For this review, take the finished solid that the model builds, in its own axes (mm). Round coordinates to 2 decimals unless told otherwise and drop trailing zeros. Order: outer loops, then holes, each group sorted by start corner. A loop starts at its lowest first (then second) coordinate and runs counter-clockwise, first axis right, second up. Notation, with made-up numbers: (38.5, 35) -> (68.5, 35) arc R17 cw to (68.5, 66) -> close; hole circle Ø8 at (-8.75, 74). An arc over 180 degrees is marked (long way). Answer in a Markdown table with one row per item.
```python
from build123d import *

# Parameters (mm, degrees)
SKETCH1_R           = 2.25
BOSS_EXTRUDE1_DEPTH = 5


with BuildPart() as part:
    # Sketch1 → Boss-Extrude1 (new body)
    with BuildSketch(Plane.XZ.offset(63)):
        with BuildLine():
            Line((8.181928414, -16.605718064), (17.802171103, -33.691169181))
            ThreePointArc((17.802171103, -33.691169181), (18.572370652, -35.426303597), (19.000782012, -37.275725803))
            ThreePointArc((19.000782012, -37.275725803), (24.55776359, -40.047666423), (25.069213931, -33.85879596))
            ThreePointArc((25.069213931, -33.85879596), (23.710027, -32.533462163), (22.625796475, -30.975148024))
            Line((22.625796475, -30.975148024), (13.005553786, -13.889696907))
            ThreePointArc((13.005553786, -13.889696907), (12.235354237, -12.15456249), (11.806942877, -10.305140285))
            ThreePointArc((11.806942877, -10.305140285), (6.249961299, -7.533199664), (5.738510958, -13.722070128))
            ThreePointArc((5.738510958, -13.722070128), (7.097697889, -15.047403925), (8.181928414, -16.605718064))
        make_face()
        with Locations((22.71787829, -36.780049236)):
            Circle(SKETCH1_R, mode=Mode.SUBTRACT)
        with Locations((8.089846599, -10.800816852)):
            Circle(SKETCH1_R, mode=Mode.SUBTRACT)
    extrude(amount=-BOSS_EXTRUDE1_DEPTH)


solid = part.part
```
Q1. The part is to be moulded in two halves that separate along X. For faces 1 (the face through (17.88, -60.54, -22.55)), 2 (the face through (7.08, -60.535, -15.027)), 3 (the face through (20.932, -60.535, -38.149)), say which applies: +X half, -X half, draft (parallel to the pull), parting line (faces both ways), or undercut.
Answer key:
| item | result |
|---|---|
| face 1 | +X half |
| face 2 | -X half |
| face 3 | undercut |
Q2. Clearance check with flat-ended pins moving along their axes: pin 1 Ø4 at (x, z) = (22, -22.5) entering from +Y; pin 2 Ø1 at (x, y) = (24, -60.5) entering from -Z. State where each tip first meets the part, or that it passes through.
Answer key:
| item | result |
|---|---|
| pin 1 | passes through |
| pin 2 | stops at z = -40.45 |
Q3. Take a section at A-A, the plane x = 9. Write out the cut boundary in (y, z).
Answer key:
| item | result |
|---|---|
| outline | (-63, -18.06) -> (-58, -18.06) -> (-58, -12.86) -> (-63, -12.86) -> close; (-63, -8.74) -> (-58, -8.74) -> (-58, -7.16) -> (-63, -7.16) -> close |
Q4. Take a section at B-B, the plane y = -61.7. Write out the cut boundary in (x, z), then the cut area to 3 significant figures.
Answer key:
| item | result |
|---|---|
| outline | (5.74, -13.72) arc R10 cw to (8.18, -16.61) -> (17.8, -33.69) arc R10 cw to (19, -37.28) arc R3.75 ccw (long way) to (25.07, -33.86) arc R10 cw to (22.63, -30.98) -> (13.01, -13.89) arc R10 cw to (11.81, -10.31) arc R3.75 ccw (long way) to start; hole circle Ø4.5 at (8.09, -10.8); hole circle Ø4.5 at (22.72, -36.78) |
| area | 186 mm^2 |
Q5. Take a section at D-D, the plane x = 17. Write out the cut boundary in (y, z).
Answer key:
| item | result |
|---|---|
| outline | (-63, -32.27) -> (-58, -32.27) -> (-58, -20.98) -> (-63, -20.98) -> close |
Q6. Take a section at C-C, the plane z = -33. Write out the cut boundary in (x, y).
Answer key:
| item | result |
|---|---|
| outline | (17.41, -63) -> (24.13, -63) -> (24.13, -58) -> (17.41, -58) -> close |
Q7. To check wall thickness, follow probe 1 along Z at (x, y) = (9.75, -61.5); probe 2 along X at (y, z) = (-61.95, -38.5); probe 3 along Z at (x, y) = (22.5, -60.95). State the ranges of each line that lie inside material, in increasing order.
Answer key:
| item | result |
|---|---|
| probe 1 | z = -19.39 to -12.32, -9.28 to -7.44 |
| probe 2 | x = 19.39 to 21.27, 24.17 to 26.05 |
| probe 3 | z = -40.52 to -39.02, -34.54 to -30.75 |
